Job drawing, mm, ordinate dimensions from the low corner. One solid piece. Coordinates: 2 decimals unless noted, no trailing zeros. Write each loop counter-clockwise with the first axis right and the second up, starting at its lowest first coordinate (ties: lowest second). Pieces come first, ordered by that corner, then holes. Notation, with made-up numbers: (-21.5, 66) - (0.5, 66) arc R25 cw to (0.5, 100) - close; hole circle Ø10 at (-33, 83.5). An arc over 180 degrees is marked (long way). Use one line per item in the form item = value. Start each with the question number.
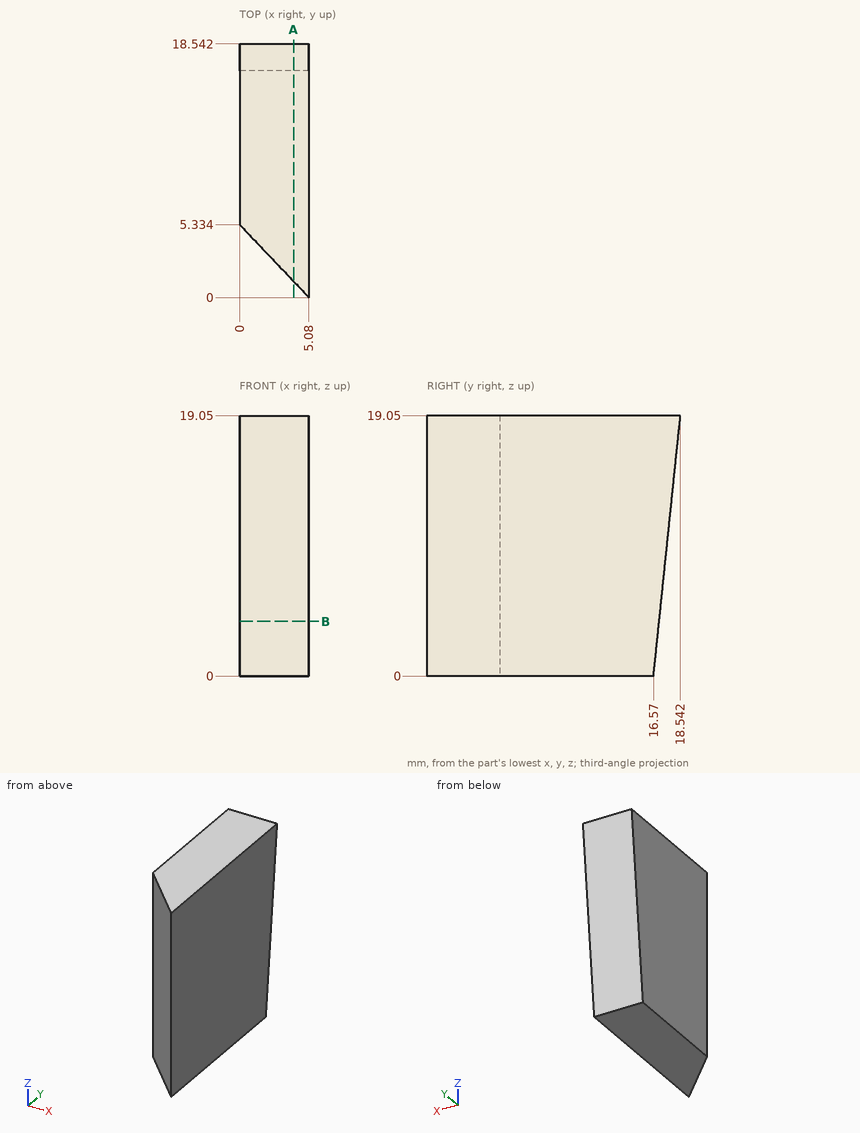
Q1. Pin check, flat tip, straight feed: P1, Ø6, axis at y = 15.5, z = 8, coming from the -X side. Stop position of the tip, or through.
Q2. Slice it at A-A (x = 3.95). List the corners of the cut face in (y, z), plus the area to 3 significant figures.
Q3. Drill centre lines: probe 1 along X at (y, z) = (2, 6.5); probe 2 along Y at (x, z) = (0.85, 16); probe 3 along Y at (x, z) = (0.6, 14.75). Where is each one in solid material? Low to high.
Q4. Slice it at B-B (z = 4). List the corners of the cut face in (x, y), plus the area to 3 significant figures.
Solution:
q1.P1 = 0
q2.outline = (1.19, 0) - (16.57, 0) - (18.54, 19.05) - (1.19, 19.05) - close
q2.area = 312 mm2
q3.probe_1 = 3.18 to 5.08
q3.probe_2 = 4.44 to 18.23
q3.probe_3 = 4.7 to 18.1
q4.outline = (0, 5.33) - (5.08, 0) - (5.08, 16.98) - (0, 16.98) - close
q4.area = 72.7 mm2
